```python
from build123d import *

# Parameters (mm, degrees)
SKETCH1_R           = 17.5
SKETCH1_R_2         = 14.5
BOSS_EXTRUDE1_DEPTH = 10
BOSS_EXTRUDE2_DEPTH = 10
SKETCH5_R           = 3
BOSS_EXTRUDE3_DEPTH = 10
FILLET1_R           = 3
SKETCH6_R           = 1.5
CUT_EXTRUDE1_DEPTH  = 10
CUT_EXTRUDE2_DEPTH  = 4


with BuildPart() as part:
    # Sketch1 → Boss-Extrude1 (new body)
    with BuildSketch(Plane.XY):
        Circle(SKETCH1_R)
        Circle(SKETCH1_R_2, mode=Mode.SUBTRACT)
    extrude(amount=BOSS_EXTRUDE1_DEPTH)

    # Sketch4 → Boss-Extrude2 (add)
    with BuildSketch(Plane.XY.offset(10)):
        Polygon((-3, 19.250821316), (-3, 16.430441273), (3, 16.430441273), (3, 19.250821316), (3, 24.327875781), (-3, 24.327875781), align=None)
    extrude(amount=-BOSS_EXTRUDE2_DEPTH)

    # Sketch5 → Boss-Extrude3 (add)
    with BuildSketch(Plane.XY.offset(10)):
        with Locations((0, 24.327875781)):
            Circle(SKETCH5_R)
    extrude(amount=-BOSS_EXTRUDE3_DEPTH)

    # Fillet1
    fillet1_edges = [part.edges().sort_by_distance(p)[0] for p in [
        (3, 17.24093965, 5),
        (-3, 17.24093965, 5),
    ]]
    fillet(fillet1_edges, radius=FILLET1_R)

    # Sketch6 → Cut-Extrude1 (cut)
    with BuildSketch(Plane.XY.offset(10)):
        with Locations((0, 24.327875781)):
            Circle(SKETCH6_R)
    extrude(amount=-CUT_EXTRUDE1_DEPTH, mode=Mode.SUBTRACT)

    # Sketch7 → Cut-Extrude2 (cut)
    with BuildSketch(Plane.XY.offset(7)):
        Polygon((-6, 21.148402448), (3.429094676, 21.148402448), (5.067314065, 21.148402448), (5.31985813, 21.327875781), (5.31985813, 28.263680706), (-6, 28.263680706), align=None)
    extrude(amount=-CUT_EXTRUDE2_DEPTH, mode=Mode.SUBTRACT)


solid = part.part
```
Geometry: final body of the model. Coordinates: model frame, mm. A direction names the side the tool comes from. Round coordinates to 2 decimals unless told otherwise and drop trailing zeros. Order: outer loops, then holes, each group sorted by start corner. A loop starts at its lowest first (then second) coordinate and runs counter-clockwise, first axis right, second up. Notation, with made-up numbers: (-27.75, -37) - (-21.75, -37) arc R10 ccw to (-21.75, -18) - close; hole circle Ø3 at (46.5, 17.5). An arc over 180 degrees is marked (long way). Use CSV: the item, a comma, the result in double quotes. Start each with the question number.
Q1. Section query A-A (y = 0). Return loops of the section in (x, z), and give its area (3 significant figures).
Q2. First-contact query: pin 1 (1.4 mm diameter, centred on y = 21, z = 3, fed in from -X); pin 2 (2 mm diameter, centred on x = 1.5, z = 5.5, fed in from +Y); pin 3 (1 mm diameter, centred on x = 9.5, z = 2, fed in from +Y); pin 4 (12 mm diameter, centred on x = -7.5, y = 1.5, fed in from -Z). Flat tips, straight axial feed; report the tip coordinate or a pass-through.
Q3. Access query for faces 1 (the face through (1, 23, 7)), 2 (the face through (0.066, 27.327, 1.521)), 3 (the face through (-3, 20.9, 5.1)), 4 (the face through (3, 20.9, 5.1)). Directions: +Z, -Z, +X, -X, +Y, -Y. A direction counts if a zero-diameter tool reaches every point of the face in a straight line with its end or side. Return the directions, or none.
Q4. Section query C-C (z = 2.5). Return loops of the section in (x, y), and give its area (3 significant figures).
Q5. Material intervals for line 1 along X through (y, z) = (-9, 5.5); line 2 along X through (y, z) = (6.5, 6.5); line 3 along Y through (x, z) = (-11.5, 1.5), sorted ascending. Write a range as from..to.
Q6. Section query B-B (x = 0). Return loops of the section in (y, z).
Q7. Mould query, pull axis X, two halves, no side actions, for faces 5 (the face through (0, 15, 0)), 6 (the face through (-3.6, 17.8, 4.9)), 7 (the face through (6.691, -12.864, 4.93)). Classes: +X half, -X half, draft (parallel to the pull), parting line (faces both ways), or undercut.
Q8. Section query D-D (z = 4.75). Return loops of the section in (x, y).
Result set:
1,outline,"(-17.5, 0) - (-14.5, 0) - (-14.5, 10) - (-17.5, 10) - close; (14.5, 0) - (17.5, 0) - (17.5, 10) - (14.5, 10) - close"
1,area,"60.0 mm2"
2,pin 1,"stops at x = -3"
2,pin 2,"stops at y = 21.15"
2,pin 3,"stops at y = 15.01"
2,pin 4,"passes through"
3,face 1,"+X, -X, +Y"
3,face 2,"+Z, -Z, +Y"
3,face 3,"+Z, -Z, -X, +Y"
3,face 4,"+Z, -Z, +X, +Y"
4,outline,"(-5.12, 16.73) arc R17.5 ccw (long way) to (5.12, 16.73) arc R3 cw to (3, 19.6) - (3, 24.33) arc R3 ccw to (-3, 24.33) - (-3, 19.6) arc R3 cw to start; hole circle Ø29 at (0, 0); hole circle Ø3 at (0, 24.33)"
4,area,"352 mm2"
5,line 1,"x = -15.01..-11.37, 11.37..15.01"
5,line 2,"x = -16.25..-12.96, 12.96..16.25"
5,line 3,"y = -13.19..-8.83, 8.83..13.19"
6,outline,"(-17.5, 0) - (-14.5, 0) - (-14.5, 10) - (-17.5, 10) - close; (14.5, 0) - (22.83, 0) - (22.83, 3) - (21.15, 3) - (21.15, 7) - (22.83, 7) - (22.83, 10) - (14.5, 10) - close; (25.83, 0) - (27.33, 0) - (27.33, 3) - (25.83, 3) - close; (25.83, 7) - (27.33, 7) - (27.33, 10) - (25.83, 10) - close"
7,face 5,"draft"
7,face 6,"-X half"
7,face 7,"undercut"
8,outline,"(-5.12, 16.73) arc R17.5 ccw (long way) to (5.12, 16.73) arc R3 cw to (3, 19.6) - (3, 21.15) - (-3, 21.15) - (-3, 19.6) arc R3 cw to start; hole circle Ø29 at (0, 0)"
